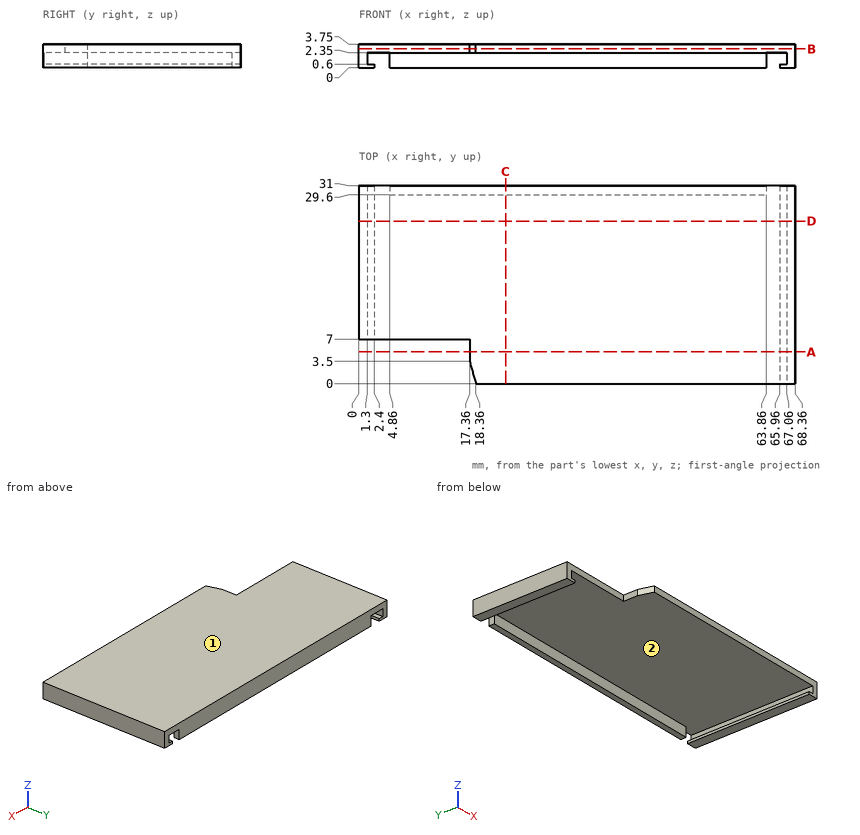
Verification items for this drawing (mm, ordinates from the low corner). Round coordinates to 2 decimals unless told otherwise and drop trailing zeros. Loops run counter-clockwise (first coordinate to the right, second up) from the corner with the lowest first, then second, coordinate; pieces in that order, holes last. Notation, with made-up numbers: (42, -21.5) -> (64, -21.5) arc R31 ccw to (64, 8.5) -> close; hole circle Ø9 at (58.25, 49.25). An arc over 180 degrees is marked (long way). Answer in a Markdown table with one row per item.
Q1. Release check for a two-part mould opening along X. For the marked faces 1 and 2 record: released by +X, released by -X, zero draft, split by the parting line, or undercut.
Data:
| item | result |
|---|---|
| face 1 | zero draft |
| face 2 | undercut |
Q2. Sectioned sample at D-D on y = 25.5. Enter the section's corners in (x, z).
Data:
| item | result |
|---|---|
| outline | (0, 0) -> (2.4, 0) -> (2.4, 0.6) -> (1.3, 0.6) -> (1.3, 2.35) -> (67.06, 2.35) -> (67.06, 0.6) -> (65.96, 0.6) -> (65.96, 0) -> (68.36, 0) -> (68.36, 3.75) -> (0, 3.75) -> close |
Q3. Thickness scan on L1, parallel to X at y = 11, z = 1.7; L2, parallel to X at y = 13, z = 0.3; L3, parallel to Y at x = 58.5, z = 0.6. Record the ranges inside material, lowest first.
Data:
| item | result |
|---|---|
| L1 | x = 0 to 1.3, 67.06 to 68.36 |
| L2 | x = 0 to 2.4, 65.96 to 68.36 |
| L3 | y = 29.6 to 31 |
Q4. Sectioned sample at B-B on z = 3. Enter the section's corners in (x, y), then the cut area to 3 significant figures.
Data:
| item | result |
|---|---|
| outline | (0, 7) -> (17.36, 7) -> (17.36, 3.5) -> (18.36, 0) -> (68.36, 0) -> (68.36, 31) -> (0, 31) -> close |
| area | 2,000 mm^2 |
Q5. Sectioned sample at C-C on x = 23. Enter the section's corners in (y, z).
Data:
| item | result |
|---|---|
| outline | (0, 2.35) -> (29.6, 2.35) -> (29.6, 0) -> (31, 0) -> (31, 3.75) -> (0, 3.75) -> close |
Q6. Sectioned sample at A-A on y = 5. Enter the section's corners in (x, z), then the cut area to 3 significant figures.
Data:
| item | result |
|---|---|
| outline | (17.36, 2.35) -> (67.06, 2.35) -> (67.06, 0.6) -> (65.96, 0.6) -> (65.96, 0) -> (68.36, 0) -> (68.36, 3.75) -> (17.36, 3.75) -> close |
| area | 75.1 mm^2 |
Q7. Go/stop test with flat-tipped pins: P1, Ø9.5, axis at x = 42.5, y = 21, coming from the -Z side; P2, Ø1.5, axis at x = 12, z = 2.5, coming from the -Y side; P3, Ø1.9, axis at x = 28, z = 1, coming from the -Y side. Record where each tip stops, or that it passes through.
Data:
| item | result |
|---|---|
| P1 | stops at z = 2.35 |
| P2 | stops at y = 7 |
| P3 | stops at y = 29.6 |
